from build123d import *

# Parameters (mm, degrees)
FILLET1_SIZE = 0.21336
FILLET2_R    = 0.21336


with BuildPart() as part:
    # Sketch4 → Revolve1 (revolve)
    with BuildSketch(Plane(origin=(0, 0, 0), x_dir=(0, 0, -1), z_dir=(1, 0, 0))):
        Polygon((3.175, -21.43125), (6.35, -21.43125), (6.35, -15.875), (-6.35, -15.875), (-6.35, -19.0754), (3.175, -19.0754), align=None)
    revolve(axis=Axis((0, 0, 6.35), (0, 0, -1)))

    # Fillet1
    fillet1_edges = [part.edges().sort_by_distance(p)[0] for p in [
        (0, 19.0754, 6.35),
        (0, 15.875, 6.35),
        (0, 15.875, -6.35),
        (0, 21.43125, -6.35),
        (0, 21.43125, -3.175),
    ]]
    chamfer(fillet1_edges, length=FILLET1_SIZE)

    # Fillet2
    fillet2_edges = [part.edges().sort_by_distance(p)[0] for p in [
        (0, 19.0754, -3.175),
    ]]
    fillet(fillet2_edges, radius=FILLET2_R)


solid = part.part
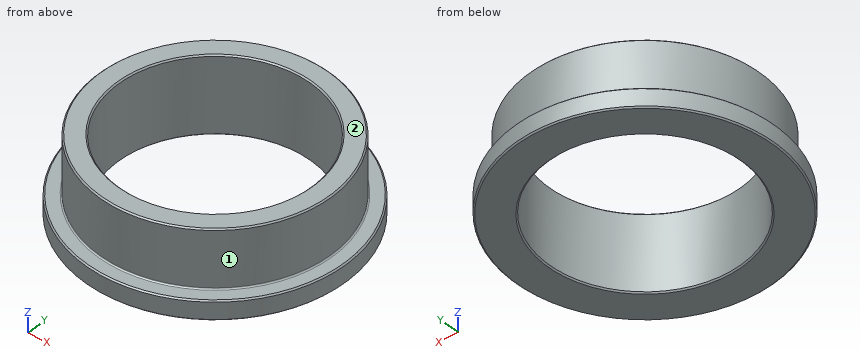
The listing builds one solid part. Answer for the finished solid, in the listing's coordinates (mm). Face numbers are marked on the shaded views. A direction names the side the tool comes from. Give positions to 0.01 mm unless a question says otherwise; leave off trailing zeros. Write each loop counter-clockwise with the first axis right and the second up, starting at its lowest first coordinate (ties: lowest second). Pieces come first, ordered by that corner, then holes.
1) A tool of negligible diameter and unlimited length cuts with its end or side. For the marked faces 1 and 2, from which of +Z, -Z, +X, -X, +Y, -Y can it reach the whole face along a straight path? Write none if from no direction.
2) Section A-A (y = 0) is taken. Write down the section's boundary in (x, z) (3 decimals), and give its area (3 significant figures).
3) Find the intervals of material crossed by L1, parallel to X at y = 0, z = 2.25 (3 decimals); L2, parallel to Y at x = 0, z = -3.5 (3 decimals), in increasing order.
4) Given P1, Ø3, axis at y = -6, z = 2.5, coming from the -X side; P2, Ø6, axis at x = 0, y = -13, coming from the +Z side; P3, Ø5, axis at x = 13.5, z = 2.5, coming from the +Y side, each flat-ended and moving along its own axis, determine where each tip first touches the part or whether it passes through.
5) Section D-D (z = 4.75) is taken. Write down the section's boundary in (x, y) (3 decimals), and give its area (3 significant figures).
Response:
1. face 1: +Z
1. face 2: +Z, +X, -X, +Y, -Y
2. outline: (-21.431, -6.137) - (-21.218, -6.35) - (-16.088, -6.35) - (-15.875, -6.137) - (-15.875, 6.137) - (-16.088, 6.35) - (-18.862, 6.35) - (-19.075, 6.137) - (-19.075, -2.962) arc R0.213 cw to (-19.289, -3.175) - (-21.218, -3.175) - (-21.431, -3.388) - close; (15.875, -6.137) - (16.088, -6.35) - (21.218, -6.35) - (21.431, -6.137) - (21.431, -3.388) - (21.218, -3.175) - (19.289, -3.175) arc R0.213 cw to (19.075, -2.962) - (19.075, 6.137) - (18.862, 6.35) - (16.088, 6.35) - (15.875, 6.137) - close
2. area: 96.0 mm2
3. L1: x = -19.075 to -15.875, 15.875 to 19.075
3. L2: y = -21.431 to -15.875, 15.875 to 21.431
4. P1: stops at x = -18.54
4. P2: stops at z = 6.26
4. P3: stops at y = 15.58
5. outline: circle Ø38.151 at (0, 0); hole circle Ø31.75 at (0, 0)
5. area: 351 mm2
